The model under review builds one solid part; all positions refer to its coordinate system, in mm. Face numbers are marked on the shaded views. A direction names the side the tool comes from. Coordinates: 2 decimals unless noted, no trailing zeros. Write each loop counter-clockwise with the first axis right and the second up, starting at its lowest first coordinate (ties: lowest second). Pieces come first, ordered by that corner, then holes. Notation, with made-up numbers: (83.5, 47.25) - (91.5, 47.25) arc R6 ccw to (91.5, 55.25) - close; hole circle Ø5 at (85, 14). An arc over 180 degrees is marked (long way). Answer as CSV lines item,"result". Start each with the question number.
```python
from build123d import *

# Parameters (mm, degrees)
SKETCH003_R             = 11.914086
PAD001_DEPTH            = 6
SKETCH004_R             = 2.55
POCKET001_DEPTH         = 74.457219
POLARPATTERN_COUNT      = 13
SKETCH062_R             = 2.575
POCKET014_DEPTH         = 1.2
BODY001_PLACEMENT_ANGLE = 90


with BuildPart() as part:
    # Sketch003 → Pad001 (new body)
    with BuildSketch(Plane.XY):
        Circle(SKETCH003_R)
        with BuildLine():
            ThreePointArc((-1.681703, 1.95), (0, -2.575), (1.681703, 1.95))
            Line((-1.681703, 1.95), (1.681703, 1.95))
        make_face(mode=Mode.SUBTRACT)
    extrude(amount=PAD001_DEPTH)

    # Sketch004 (on Face5 of Pad001) → Pocket001 (cut, through all)
    with BuildSketch(Plane.XY.offset(6)):
        with Locations((0, 12.414086)):
            Circle(SKETCH004_R)
    pocket001 = extrude(amount=-POCKET001_DEPTH, mode=Mode.SUBTRACT)

    # PolarPattern: Pocket001 ×13 about axis
    polarpattern_axis = Axis((0, 0, 6), (0, 0, 1))
    for i in range(1, POLARPATTERN_COUNT):
        add(pocket001.rotate(polarpattern_axis, i * 360 / POLARPATTERN_COUNT), mode=Mode.SUBTRACT)

    # Sketch062 (on Face4 of PolarPattern) → Pocket014 (cut)
    with BuildSketch(Plane.XY.offset(6)):
        Circle(SKETCH062_R)
    extrude(amount=-POCKET014_DEPTH, mode=Mode.SUBTRACT)


with BuildPart() as part_1:
    # Body001 placement: moved
    add(part.part.moved(Location((-5.85, -50.15, 2.4))).rotate(Axis((-5.85, -50.15, 2.4), (0, 0, 1)), BODY001_PLACEMENT_ANGLE))


solid = part_1.part
```
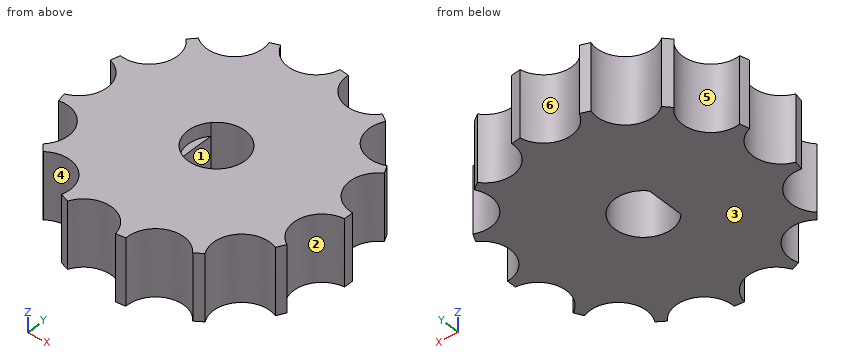
(1) For the marked faces 1 and 2, list the 3-axis set-ups (+Z, -Z, +X, -X, +Y, -Y) from which the entire face can be reached by the end or side of a thin tool; tool diameter is ignored.
(2) Add section B-B on y = -51.5. Give the boundary of the cut face in (x, z).
(3) Wall thickness on line 1 (X direction, y = -50.15, z = 5.65) (3 decimals); line 2 (Y direction, x = -14.75, z = 8.15); line 3 (Y direction, x = -5.85, z = 6.95) (3 decimals): over which ranges is each line inside the solid? List them lowest first.
(4) Add section D-D on x = -12.75. Give the boundary of the cut face in (y, z).
(5) The part is to be moulded in two halves that separate along Y. For the marked faces 3, 4, 5 and 6, say which applies: released by +Y, released by -Y, zero draft, split by the parting line, or undercut.
(6) Add section C-C on x = -5.85. Give the boundary of the cut face in (y, z) (3 decimals), then the cut area to 3 significant figures.
(7) For pin 1 (1.5 mm diameter, centred on x = -3.5, z = 4, fed in from +Y); pin 2 (2 mm diameter, centred on x = -1.5, z = 3, fed in from -Y), all flat-tipped, find the tip position at first contact; note any pin that passes through.
Reported:
1,face 1,"+Z, -Z"
1,face 2,"+Z, -Z, +X"
2,outline,"(-16.1, 2.4) - (-7.8, 2.4) - (-7.8, 7.2) - (-8.04, 7.2) - (-8.04, 8.4) - (-16.1, 8.4) - close; (-3.66, 2.4) - (4.23, 2.4) - (4.23, 8.4) - (-3.66, 8.4) - close"
3,line 1,"-15.714 to -7.8, -3.275 to 6.064"
3,line 2,"-58.07 to -57.38, -54.46 to -45.84, -42.92 to -42.23"
3,line 3,"-60.409 to -52.725, -47.575 to -39.891"
4,outline,"(-57.82, 2.4) - (-42.48, 2.4) - (-42.48, 8.4) - (-57.82, 8.4) - close"
5,face 3,"zero draft"
5,face 4,"undercut"
5,face 5,"undercut"
5,face 6,"released by +Y"
6,outline,"(-60.409, 2.4) - (-52.725, 2.4) - (-52.725, 8.4) - (-60.409, 8.4) - close; (-47.575, 2.4) - (-39.891, 2.4) - (-39.891, 8.4) - (-47.575, 8.4) - close"
6,area,"92.2 mm²"
7,pin 1,"y = -38.34"
7,pin 2,"y = -59.43"
